Geometry: final body of the model. Coordinates: model frame, mm. Face numbers are marked on the shaded views. A direction names the side the tool comes from. Round coordinates to 2 decimals unless told otherwise and drop trailing zeros. Order: outer loops, then holes, each group sorted by start corner. A loop starts at its lowest first (then second) coordinate and runs counter-clockwise, first axis right, second up. Notation, with made-up numbers: M 36.5,-2.5 L 43.5,-2.5 A25 ccw 43.5,27.5 Z; hole C 56.5,29 d3. An arc over 180 degrees is marked long. Put each result on its own line as item: value. Start each with the question number.
1) Access query for the marked faces 1 and 2. Directions: +Z, -Z, +X, -X, +Y, -Y. A direction counts if a zero-diameter tool reaches every point of the face in a straight line with its end or side. Return the directions, or none.
2) Material intervals for probe 1 along Y at (x, z) = (40, 62.4); probe 2 along Y at (x, z) = (-3.5, 5.5); probe 3 along X at (y, z) = (-17, 55), sorted ascending. Write a range as [from, to].
3) Section B-B, the plane z = 37.5. Return loops of the section in (x, y), then the cut area to 3 significant figures.
4) Draft query along X for the marked faces 3, 4, 5 and 6. Return one class per face: pulls with the +X half, pulls with the -X half, needs draft (parallel to the pull), parting line crosses it, or undercut.
5) First-contact query: P1, Ø8, axis at y = -12, z = 32, coming from the +X side; P2, Ø2.5, axis at y = 16.5, z = 2, coming from the -X side; P3, Ø1.5, axis at x = -33, z = 58, coming from the -Y side. Flat tips, straight axial feed; report the tip coordinate or a pass-through.
6) Section C-C, the plane z = 20. Return loops of the section in (x, y), then the cut area to 3 significant figures.
7) Section A-A, the plane y = -3.5. Return loops of the section in (x, z), then the cut area to 3 significant figures.
8) Section D-D, the plane z = 26.5. Return loops of the section in (x, y).
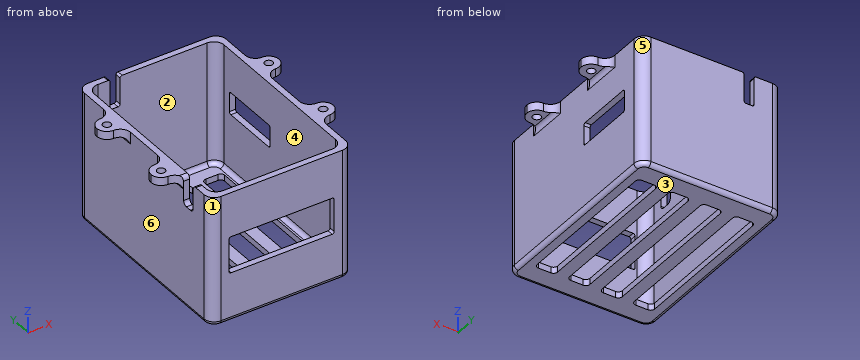
from build123d import *

# Parameters (mm, degrees)
SKETCH1_W           = 64
SKETCH1_H           = 92.29356787
SKETCH1_W_2         = 10
SKETCH1_H_2         = 76.29356787
BOSS_EXTRUDE1_DEPTH = 3
SKETCH1_3_W         = 70
SKETCH1_3_H         = 98.29356787
SKETCH1_3_W_2       = 64
SKETCH1_3_H_2       = 92.29356787
BOSS_EXTRUDE2_DEPTH = 64
FILLET1_R           = 2
FILLET2_R           = 5
SKETCH2_W           = 52
SKETCH2_H           = 18
CUT_EXTRUDE1_DEPTH  = 64
FILLET3_R           = 1
SKETCH3_W           = 11
SKETCH3_H           = 30
CUT_EXTRUDE2_DEPTH  = 45
FILLET4_R           = 1
SKETCH4_W           = 5
SKETCH4_H           = 15
CUT_EXTRUDE3_DEPTH  = 81
FILLET5_R           = 1
SKETCH5_W           = 10
SKETCH5_H           = 10
SKETCH5_R           = 2
BOSS_EXTRUDE3_DEPTH = 4
FILLET6_R           = 5
FILLET7_R           = 5
FILLET8_R           = 2
FILLET9_R           = 2
FILLET10_R          = 2
SKETCH6_W           = 13.6
SKETCH6_H           = 7
CUT_EXTRUDE4_DEPTH  = 48
FILLET11_R          = 2


with BuildPart() as part:
    # Sketch1 → Boss-Extrude1 (new body)
    with BuildSketch(Plane.XY):
        Rectangle(SKETCH1_W, SKETCH1_H)
        with Locations((-24, 0)):
            Rectangle(SKETCH1_W_2, SKETCH1_H_2, mode=Mode.SUBTRACT)
        with Locations((-8, 0)):
            Rectangle(SKETCH1_W_2, SKETCH1_H_2, mode=Mode.SUBTRACT)
        with Locations((8, 0)):
            Rectangle(SKETCH1_W_2, SKETCH1_H_2, mode=Mode.SUBTRACT)
        with Locations((24, 0)):
            Rectangle(SKETCH1_W_2, SKETCH1_H_2, mode=Mode.SUBTRACT)
    extrude(amount=BOSS_EXTRUDE1_DEPTH)

    # Sketch1<3> → Boss-Extrude2 (add)
    with BuildSketch(Plane.XY):
        Rectangle(SKETCH1_3_W, SKETCH1_3_H)
        Rectangle(SKETCH1_3_W_2, SKETCH1_3_H_2, mode=Mode.SUBTRACT)
    extrude(amount=BOSS_EXTRUDE2_DEPTH)

    # Fillet1
    fillet1_edges = [part.edges().sort_by_distance(p)[0] for p in [
        (-19, -38.146783935, 1.5),
        (-19, 38.146783935, 1.5),
        (-29, 38.146783935, 1.5),
        (-29, -38.146783935, 1.5),
        (-13, 38.146783935, 1.5),
        (-13, -38.146783935, 1.5),
        (-3, -38.146783935, 1.5),
        (-3, 38.146783935, 1.5),
        (3, 38.146783935, 1.5),
        (3, -38.146783935, 1.5),
        (13, -38.146783935, 1.5),
        (13, 38.146783935, 1.5),
        (19, 38.146783935, 1.5),
        (19, -38.146783935, 1.5),
        (29, -38.146783935, 1.5),
        (29, 38.146783935, 1.5),
    ]]
    fillet(fillet1_edges, radius=FILLET1_R)

    # Fillet2
    fillet2_edges = [part.edges().sort_by_distance(p)[0] for p in [
        (32, -46.146783935, 33.5),
        (-32, -46.146783935, 33.5),
        (-32, 46.146783935, 33.5),
        (-35, 49.146783935, 32),
        (-35, -49.146783935, 32),
        (35, -49.146783935, 32),
        (35, 49.146783935, 32),
        (32, 46.146783935, 33.5),
    ]]
    fillet(fillet2_edges, radius=FILLET2_R)

    # Sketch2 → Cut-Extrude1 (cut)
    with BuildSketch(Plane(origin=(0, 0, 0), x_dir=(1, 0, 0), z_dir=(0, 1, 0))):
        with Locations((0, -33)):
            Rectangle(SKETCH2_W, SKETCH2_H)
    extrude(amount=-CUT_EXTRUDE1_DEPTH, mode=Mode.SUBTRACT)

    # Fillet3
    fillet3_edges = [part.edges().sort_by_distance(p)[0] for p in [
        (-26, -47.646783935, 42),
        (-26, -47.646783935, 24),
        (26, -47.646783935, 24),
        (26, -47.646783935, 42),
    ]]
    fillet(fillet3_edges, radius=FILLET3_R)

    # Sketch3 → Cut-Extrude2 (cut)
    with BuildSketch(Plane(origin=(0, 0, 0), x_dir=(0, 0, -1), z_dir=(1, 0, 0))):
        with Locations((-37.5, 22.146783935)):
            Rectangle(SKETCH3_W, SKETCH3_H)
    extrude(amount=CUT_EXTRUDE2_DEPTH, mode=Mode.SUBTRACT)

    # Fillet4
    fillet4_edges = [part.edges().sort_by_distance(p)[0] for p in [
        (33.5, 37.146783935, 43),
        (33.5, 7.146783935, 43),
        (33.5, 7.146783935, 32),
        (33.5, 37.146783935, 32),
    ]]
    fillet(fillet4_edges, radius=FILLET4_R)

    # Sketch4 → Cut-Extrude3 (cut)
    with BuildSketch(Plane(origin=(0, 0, 0), x_dir=(1, 0, 0), z_dir=(0, 1, 0))):
        with Locations((-18.5, -56.5)):
            Rectangle(SKETCH4_W, SKETCH4_H)
    extrude(amount=CUT_EXTRUDE3_DEPTH, mode=Mode.SUBTRACT)

    # Fillet5
    fillet5_edges = [part.edges().sort_by_distance(p)[0] for p in [
        (-16, 47.646783935, 64),
        (-21, 47.646783935, 64),
        (-16, 47.646783935, 49),
        (-21, 47.646783935, 49),
    ]]
    fillet(fillet5_edges, radius=FILLET5_R)

    # Sketch5 → Boss-Extrude3 (add)
    # profile 1 of 4: a face of its own
    with BuildSketch(Plane.XY.offset(64)):
        with Locations((40, 20)):
            Rectangle(SKETCH5_W, SKETCH5_H)
        with Locations((40, 20)):
            Circle(SKETCH5_R, mode=Mode.SUBTRACT)
    # profile 2 of 4: a face of its own
    with BuildSketch(Plane.XY.offset(64)):
        with Locations((40, -20)):
            Rectangle(SKETCH5_W, SKETCH5_H)
        with Locations((40, -20)):
            Circle(SKETCH5_R, mode=Mode.SUBTRACT)
    # profile 3 of 4: a face of its own
    with BuildSketch(Plane.XY.offset(64)):
        with Locations((-40, -20)):
            Rectangle(SKETCH5_W, SKETCH5_H)
        with Locations((-40, -20)):
            Circle(SKETCH5_R, mode=Mode.SUBTRACT)
    # profile 4 of 4: a face of its own
    with BuildSketch(Plane.XY.offset(64)):
        with Locations((-40, 20)):
            Rectangle(SKETCH5_W, SKETCH5_H)
        with Locations((-40, 20)):
            Circle(SKETCH5_R, mode=Mode.SUBTRACT)
    extrude(amount=-BOSS_EXTRUDE3_DEPTH)

    # Fillet6
    fillet6_edges = [part.edges().sort_by_distance(p)[0] for p in [
        (35, 15, 62),
        (35, 25, 62),
        (35, -25, 62),
        (35, -15, 62),
        (-35, -15, 62),
        (-35, -25, 62),
        (-35, 25, 62),
        (-35, 15, 62),
    ]]
    fillet(fillet6_edges, radius=FILLET6_R)

    # Fillet7
    fillet7_edges = [part.edges().sort_by_distance(p)[0] for p in [
        (-45, 25, 62),
        (-45, 15, 62),
        (-45, -15, 62),
        (-45, -25, 62),
        (45, -25, 62),
        (45, -15, 62),
        (45, 15, 62),
        (45, 25, 62),
    ]]
    fillet(fillet7_edges, radius=FILLET7_R - 0.0001)  # a hair under: the kernel refuses the full size

    # Fillet8
    fillet8_edges = [part.edges().sort_by_distance(p)[0] for p in [
        (35, 20, 60),
        (35, -20, 60),
        (-35, -20, 60),
        (-35, 20, 60),
    ]]
    fillet(fillet8_edges, radius=FILLET8_R)

    # Fillet9
    fillet9_edges = [part.edges().sort_by_distance(p)[0] for p in [
        (35, 0, 0),
        (-35, 0, 0),
        (0, 49.146783935, 0),
        (0, -49.146783935, 0),
        (-33.535533906, 47.68231784, 0),
        (33.535533906, 47.68231784, 0),
        (-33.535533906, -47.68231784, 0),
        (33.535533906, -47.68231784, 0),
    ]]
    fillet(fillet9_edges, radius=FILLET9_R)

    # Fillet10
    fillet10_edges = [part.edges().sort_by_distance(p)[0] for p in [
        (-32, 0, 3),
        (0, -46.146783935, 3),
        (32, 0, 3),
        (0, 46.146783935, 3),
        (30.535533906, 44.68231784, 3),
        (-30.535533906, 44.68231784, 3),
        (30.535533906, -44.68231784, 3),
        (-30.535533906, -44.68231784, 3),
    ]]
    fillet(fillet10_edges, radius=FILLET10_R)

    # Sketch6 → Cut-Extrude4 (cut)
    with BuildSketch(Plane(origin=(0, 0, 0), x_dir=(0, 0, -1), z_dir=(1, 0, 0))):
        with Locations((-57.2, -32.646783935)):
            Rectangle(SKETCH6_W, SKETCH6_H)
    extrude(amount=-CUT_EXTRUDE4_DEPTH, mode=Mode.SUBTRACT)

    # Fillet11
    fillet11_edges = [part.edges().sort_by_distance(p)[0] for p in [
        (-33.5, -29.146783935, 50.4),
        (-33.5, -36.146783935, 50.4),
        (-33.5, -36.146783935, 64),
        (-33.536667788, -29.146783935, 64),
    ]]
    fillet(fillet11_edges, radius=FILLET11_R)


solid = part.part
Result sheet:
1. face 1: +Z, -Z, -X, -Y
1. face 2: +Z
2. probe 1: y = [-25, -22], [-18, -15], [15, 18], [22, 25]
2. probe 2: y = [-49.15, -46.15], [46.15, 49.15]
2. probe 3: x = [-35, -32], [32, 35]
3. outline: M -35,-44.15 A5 ccw -30,-49.15 L -26,-49.15 L -26,-46.15 L -27,-46.15 A5 cw -32,-41.15 L -32,41.15 A5 cw -27,46.15 L 27,46.15 A5 cw 32,41.15 L 32,37.15 L 35,37.15 L 35,44.15 A5 ccw 30,49.15 L -30,49.15 A5 ccw -35,44.15 Z; M 26,-49.15 L 30,-49.15 A5 ccw 35,-44.15 L 35,7.15 L 32,7.15 L 32,-41.15 A5 cw 27,-46.15 L 26,-46.15 Z
3. area: 728 mm2
4. face 3: needs draft
4. face 4: undercut
4. face 5: pulls with the +X half
4. face 6: pulls with the -X half
5. P1: stops at x = 35
5. P2: stops at x = -35
5. P3: stops at y = -48.61
6. outline: M -35,-44.15 A5 ccw -30,-49.15 L 30,-49.15 A5 ccw 35,-44.15 L 35,44.15 A5 ccw 30,49.15 L -30,49.15 A5 ccw -35,44.15 Z; hole M -32,-41.15 A5 ccw -27,-46.15 L 27,-46.15 A5 ccw 32,-41.15 L 32,41.15 A5 ccw 27,46.15 L -27,46.15 A5 ccw -32,41.15 Z
6. area: 974 mm2
7. outline: M -35,2 A2 ccw -33,0 L -29,0 L -29,3 L -30,3 A2 cw -32,5 L -32,64 L -35,64 Z; M -19,0 L -13,0 L -13,3 L -19,3 Z; M -3,0 L 3,0 L 3,3 L -3,3 Z; M 13,0 L 19,0 L 19,3 L 13,3 Z; M 29,0 L 33,0 A2 ccw 35,2 L 35,64 L 32,64 L 32,5 A2 cw 30,3 L 29,3 Z
7. area: 456 mm2
8. outline: M -35,-44.15 A5 ccw -30,-49.15 L -26,-49.15 L -26,-46.15 L -27,-46.15 A5 cw -32,-41.15 L -32,41.15 A5 cw -27,46.15 L 27,46.15 A5 cw 32,41.15 L 32,-41.15 A5 cw 27,-46.15 L 26,-46.15 L 26,-49.15 L 30,-49.15 A5 ccw 35,-44.15 L 35,44.15 A5 ccw 30,49.15 L -30,49.15 A5 ccw -35,44.15 Z
